The listing builds one solid part. Answer for the finished solid, in the listing's coordinates (mm). A direction names the side the tool comes from. Coordinates: 2 decimals unless noted, no trailing zeros. Order: outer loops, then holes, each group sorted by start corner. A loop starts at its lowest first (then second) coordinate and runs counter-clockwise, first axis right, second up.
from build123d import *

# Parameters (mm, degrees)
F1_DEPTH = 25


# Not quite as in the source:
# - a feature of the source that left no trace in its solid (it failed there, or was rolled back) is left out


with BuildPart() as f1:
    # F0 (on Right) → F1 (new body, symmetric)
    with BuildSketch(Plane.YZ):
        with BuildLine():
            Line((-10, 28.3795828863), (-10, 0))
            Line((-10, 0), (10, 0))
            Line((10, 0), (10, 45))
            Line((10, 45), (-150.503690731, 32.3680855878))
            add(Edge.make_bspline(
                [(-150.503690731, 32.3680855878), (-251.6470152481, 24.4079333144), (-248.2635080814, 20.058169961), (-256.3765901785, 10.171615941)],
                knots=[0, 0, 0, 0, 108.1746463003, 108.1746463003, 108.1746463003, 108.1746463003], degree=3))
            ThreePointArc((-256.3765901785, 10.171615941), (-246.5433476591, -20.3637900829), (-214.7508155307, -16.0814332135))
            add(Edge.make_bspline(
                [(-214.7508155307, -16.0814332135), (-193.5426698765, 4.8777479678), (-161.3064821603, -3.4644254483), (-134.6062239053, -11.7416404626)],
                knots=[0, 0, 0, 0, 80.2620045097, 80.2620045097, 80.2620045097, 80.2620045097], degree=3))
            Line((-134.6062239053, -11.7416404626), (-138.6023360516, 18.2583595374))
            Line((-138.6023360516, 18.2583595374), (-10, 28.3795828863))
        make_face()
    extrude(amount=F1_DEPTH, both=True)


solid = f1.part
1) Section B-B (y = -58.5) is taken. Give the vertices of the cut face in (x, z), then the cut area to 3 significant figures.
2) Determine the mould class of faces 1 (the face through (0.35, -246.95, -20.1)), 2 (the face through (0.35, -75.2, 23.25)), 3 (the face through (-25, -156, 11)) for opening direction Y: released by +Y, released by -Y, zero draft, split by the parting line, or undercut.
3) Section A-A (z = 39.5) is taken. Give the vertices of the cut face in (x, y), then the cut area to 3 significant figures.
4) Each of these flat-tipped pins is pushed along its axis until it touches: P1, Ø1, axis at x = 6.5, y = -204.5, coming from the +Z side; P2, Ø12, axis at x = 0, y = -149, coming from the +Z side; P3, Ø1.5, axis at x = 18.5, z = -0.5, coming from the -Y side. Where does it stop, or does it pass through?
5) Consider L1, parallel to Y at x = -6.5, z = 14; L2, parallel to Z at x = -15, y = -19.5; L3, parallel to Z at x = -20, y = -78.5. Determine where each line is inside the solid, lowest interval first.
6) A tool of negligible diameter and unlimited length cuts with its end or side. For faces 4 (the face through (0, 10, 22)), 5 (the face through (0.35, -136.576, 3.048)), 6 (the face through (25, -156, 11)), 7 (the face through (0, -10, 14)), 8 (the face through (0, 0, 0)), from which of +Z, -Z, +X, -X, +Y, -Y can it reach the whole face along a straight path? Write none if from no direction.
Filled sheet:
1. outline: (-25, 24.56) - (25, 24.56) - (25, 39.61) - (-25, 39.61) - close
1. area: 752 mm2
2. face 1: split by the parting line
2. face 2: undercut
2. face 3: zero draft
3. outline: (-25, -59.88) - (25, -59.88) - (25, 10) - (-25, 10) - close
3. area: 3,490 mm2
4. P1: stops at z = 27.46
4. P2: stops at z = 32.96
4. P3: stops at y = -258.2
5. L1: y = -253.35 to -138.04, -10 to 10
5. L2: z = 27.63 to 42.68
5. L3: z = 22.99 to 38.03
6. face 4: +Z, -Z, +X, -X, +Y
6. face 5: +X, -X
6. face 6: +Z, -Z, +X, +Y, -Y
6. face 7: -Z, +X, -X
6. face 8: -Z, +X, -X, +Y
